```python
from build123d import *

# Parameters (mm, degrees)
SKETCH1_R           = 2.45
BOSS_EXTRUDE1_DEPTH = 4.5
SKETCH2_R           = 2.375
CUT_EXTRUDE1_DEPTH  = 5.5


with BuildPart() as part:
    # Sketch1 → Boss-Extrude1 (new body)
    with BuildSketch(Plane(origin=(0, 0, 0), x_dir=(1, 0, 0), z_dir=(0, 1, 0))):
        Polygon((27.15, 26), (37.15, 16), (37.15, 10), (27.15, 0), (-27.15, 0), (-37.15, 10), (-37.15, 16), (-27.15, 26), align=None)
        with Locations((24.8, 13)):
            Circle(SKETCH1_R, mode=Mode.SUBTRACT)
        with Locations((-24.8, 13)):
            Circle(SKETCH1_R, mode=Mode.SUBTRACT)
    extrude(amount=BOSS_EXTRUDE1_DEPTH)

    # Sketch2 → Cut-Extrude1 (cut, through all)
    with BuildSketch(Plane(origin=(0, 4.5, 0), x_dir=(1, 0, 0), z_dir=(0, 1, 0))):
        with Locations((3.5, 13)):
            Circle(SKETCH2_R)
    extrude(amount=-CUT_EXTRUDE1_DEPTH, mode=Mode.SUBTRACT)


solid = part.part
```
Design review of the part built by this model. Coordinates are the model's own, in mm. Round coordinates to 2 decimals unless told otherwise and drop trailing zeros. Order: outer loops, then holes, each group sorted by start corner. A loop starts at its lowest first (then second) coordinate and runs counter-clockwise, first axis right, second up. Notation, with made-up numbers: (-38.5, 74.25) - (-25.5, 74.25) arc R21 cw to (-25.5, 95.25) - close; hole circle Ø1 at (16.5, 51). An arc over 180 degrees is marked (long way). One line per question, with ' | ' between items.
Item 1: Take a section at B-B, the plane x = 3.5. Write out the cut boundary in (y, z) (3 decimals), then the cut area to 3 significant figures.
Checks:
outline: (0, -26) - (4.5, -26) - (4.5, -15.375) - (0, -15.375) - close; (0, -10.625) - (4.5, -10.625) - (4.5, 0) - (0, 0) - close | area: 95.6 mm²
Item 2: Take a section at C-C, the plane y = 3.15. Write out the cut boundary in (x, z) (3 decimals).
Checks:
outline: (-37.15, -16) - (-27.15, -26) - (27.15, -26) - (37.15, -16) - (37.15, -10) - (27.15, 0) - (-27.15, 0) - (-37.15, -10) - close; hole circle Ø4.9 at (-24.8, -13); hole circle Ø4.75 at (3.5, -13); hole circle Ø4.9 at (24.8, -13)
Item 3: Wall thickness on line 1 (X direction, y = 2.7, z = -13) (3 decimals); line 2 (Z direction, x = -24.8, y = 1.35); line 3 (Z direction, x = -23, y = 0.75): over which ranges is each line inside the solid? List them lowest first. Write a range as [from, to].
Checks:
line 1: [-37.15, -27.25], [-22.35, 1.125], [5.875, 22.35], [27.25, 37.15] | line 2: [-26, -15.45], [-10.55, 0] | line 3: [-26, -14.66], [-11.34, 0]
Item 4: For P1, Ø8, axis at x = 24.8, z = -13, coming from the -Y side; P2, Ø1.5, axis at y = 1, z = -20, coming from the +X side, all flat-tipped, find the tip position at first contact; note any pin that passes through.
Checks:
P1: y = 0 | P2: x = 33.9
Item 5: Take a section at A-A, the plane z = -13. Write out the cut boundary in (x, y) (3 decimals), then the cut area to 3 significant figures.
Checks:
outline: (-37.15, 0) - (-27.25, 0) - (-27.25, 4.5) - (-37.15, 4.5) - close; (-22.35, 0) - (1.125, 0) - (1.125, 4.5) - (-22.35, 4.5) - close; (5.875, 0) - (22.35, 0) - (22.35, 4.5) - (5.875, 4.5) - close; (27.25, 0) - (37.15, 0) - (37.15, 4.5) - (27.25, 4.5) - close | area: 269 mm²
Item 6: Draft analysis for pull direction Z (two halves, no side actions). For faces 1 (the face through (-37.15, 2, -13)), 2 (the face through (-22.463, 2.218, -13.736)), 3 (the face through (32.22, 2.22, -5.07)), 4 (the face through (0, 2, -26)), state which applies: +Z half, -Z half, draft (parallel to the pull), parting line (faces both ways), or undercut.
Checks:
face 1: draft | face 2: undercut | face 3: +Z half | face 4: -Z half
Item 7: Take a section at D-D, the plane x = -24.8. Write out the cut boundary in (y, z).
Checks:
outline: (0, -26) - (4.5, -26) - (4.5, -15.45) - (0, -15.45) - close; (0, -10.55) - (4.5, -10.55) - (4.5, 0) - (0, 0) - close
